```python
from build123d import *

# Parameters (mm, degrees)
BOSS_EXTRUDE1_DEPTH = 3.175
FILLET1_R           = 6.35
SKETCH2_R           = 2.032
SKETCH2_R_2         = 1.778
CUT_EXTRUDE1_DEPTH  = 24.8917433


with BuildPart() as part:
    # Sketch1 → Boss-Extrude1 (new body)
    with BuildSketch(Plane(origin=(0, 0, 0), x_dir=(1, 0, 0), z_dir=(0, 1, 0))):
        with BuildLine():
            Line((-8.468627029, -13.126027192), (0, -3.175))
            Line((0, -3.175), (8.468627029, -13.126027192))
            ThreePointArc((8.468627029, -13.126027192), (17.244713502, -12.721481385), (14.65849127, -4.325362897))
            Line((14.65849127, -4.325362897), (3.175, 0))
            Line((3.175, 0), (14.65849127, 4.325362897))
            ThreePointArc((14.65849127, 4.325362897), (17.244713502, 12.721481385), (8.468627029, 13.126027192))
            Line((8.468627029, 13.126027192), (0, 3.175))
            Line((0, 3.175), (-8.468627029, 13.126027192))
            ThreePointArc((-8.468627029, 13.126027192), (-17.244713502, 12.721481385), (-14.65849127, 4.325362897))
            Line((-14.65849127, 4.325362897), (-3.175, 0))
            Line((-3.175, 0), (-14.65849127, -4.325362897))
            ThreePointArc((-14.65849127, -4.325362897), (-17.244713502, -12.721481385), (-8.468627029, -13.126027192))
        make_face()
    extrude(amount=BOSS_EXTRUDE1_DEPTH)

    # Fillet1
    fillet1_edges = [part.edges().sort_by_distance(p)[0] for p in [
        (0, 1.5875, -3.175),
        (-3.175, 1.5875, 0),
        (3.175, 1.5875, 0),
        (0, 1.5875, 3.175),
    ]]
    fillet(fillet1_edges, radius=FILLET1_R)

    # Sketch2 → Cut-Extrude1 (cut, through all)
    with BuildSketch(Plane(origin=(0, 3.175, 0), x_dir=(1, 0, 0), z_dir=(0, 1, 0))):
        with Locations(Location((-12.7, 9.525, 0), (0, 0, 270))):
            Circle(SKETCH2_R)
        with Locations(Location((12.7, 9.525, 0), (0, 0, 270))):
            Circle(SKETCH2_R)
        with Locations(Location((12.7, -9.525, 0), (0, 0, 270))):
            Circle(SKETCH2_R)
        with Locations(Location((-12.7, -9.525, 0), (0, 0, 270))):
            Circle(SKETCH2_R_2)
    extrude(amount=-CUT_EXTRUDE1_DEPTH, mode=Mode.SUBTRACT)


solid = part.part
```
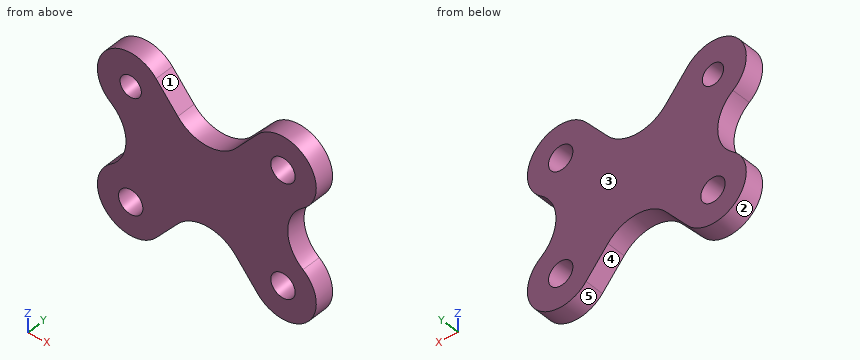
Read the model definition and answer for the solid it produces. Units are mm, in the model's axes. Face numbers are marked on the shaded views. A direction names the side the tool comes from. Give positions to 0.01 mm unless a question says otherwise; leave off trailing zeros. Order: outer loops, then holes, each group sorted by start corner. A loop starts at its lowest first (then second) coordinate and runs counter-clockwise, first axis right, second up.
(1) For the marked faces 1 and 2, determine the directions among +Z, -Z, +X, -X, +Y, -Y from which every point of the face is accessible in a straight line to the end or side of a thin tool.
(2) Given pin 1 (3.5 mm diameter, centred on x = -12.7, z = -9.525, fed in from -Y), flat-ended and moving along its own axis, determine where the tip first touches the part or whether it passes through.
(3) Find section C-C (x = 12.7). Give the vertices of the cut face in (y, z) (3 decimals).
(4) Find section D-D (y = 0.5). Give the number of separate pieces and of enclosed holes in the cut face, plus the area to 3 significant figures.
(5) Find section A-A (x = -12.7). Give the vertices of the cut face in (y, z) (3 decimals), plus the area to 3 significant figures.
(6) Find section B-B (z = 12.5). Give the vertices of the cut face in (x, y) (3 decimals).
(7) Straight lines are drawn through the part: L1, parallel to X at y = 1.1, z = 8; L2, parallel to X at y = 2.15, z = -9.5; L3, parallel to X at y = 1.15, z = 0. For each, find the intervals that lie inside material, in ascending order.
(8) For a pull along Z with two mould halves and no side action, classify the marked faces 3, 4 and 5 as released by +Z, released by -Z, zero draft, split by the parting line, or undercut.
Result sheet:
1. face 1: +Z, +Y, -Y
1. face 2: +Y, -Y
2. pin 1: passes through
3. outline: (0, -15.081) - (3.175, -15.081) - (3.175, -11.557) - (0, -11.557) - close; (0, -7.493) - (3.175, -7.493) - (3.175, 7.493) - (0, 7.493) - close; (0, 11.557) - (3.175, 11.557) - (3.175, 15.081) - (0, 15.081) - close
4. separate pieces: 1
4. enclosed holes: 4
4. area: 713 mm2
5. outline: (0, -15.081) - (3.175, -15.081) - (3.175, -11.557) - (0, -11.557) - close; (0, -7.493) - (3.175, -7.493) - (3.175, 7.747) - (0, 7.747) - close; (0, 11.303) - (3.175, 11.303) - (3.175, 15.081) - (0, 15.081) - close
5. area: 71.6 mm2
6. outline: (-17.393, 0) - (-7.936, 0) - (-7.936, 3.175) - (-17.393, 3.175) - close; (7.936, 0) - (17.393, 0) - (17.393, 3.175) - (7.936, 3.175) - close
7. L1: x = -18.04 to -13.61, -11.79 to -3.95, 3.95 to 11.36, 14.04 to 18.04
7. L2: x = -18.26 to -14.73, -10.67 to -5.38, 5.38 to 10.67, 14.73 to 18.26
7. L3: x = -13.49 to 13.49
8. face 3: zero draft
8. face 4: released by -Z
8. face 5: undercut
